Autodesk Inventor part; units mm, degrees
ref_plane "YZ Plane" through (0, 0, 0) normal (1, 0, 0) x (0, 1, 0)
ref_plane "XZ Plane" through (0, 0, 0) normal (0, 1, 0) x (-1, 0, 0)
ref_plane "XY Plane" through (0, 0, 0) normal (0, 0, 1) x (1, 0, 0)
sketch "Boceto1" plane through (0, 0, 0) normal (0, 1, 0) x (-1, 0, 0)
  line L0 (50, 50) -> (-50, 50)
  line L1 (-50, 50) -> (-50, -50)
  line L2 (-50, -50) -> (50, -50)
  line L3 (50, -50) -> (50, 50)
  line L4 (50, 50) -> (-50, -50) construction
  line L5 (-50, 50) -> (50, -50) construction
  point P0 (0, 0)
  dimension "d0" = 100
  dimension "d1" = 100
extrude "Extrusión1" add sketch "Boceto1" along normal blind 10
sketch "Boceto2" plane through (0, 10, 0) normal (0, 1, 0) x (1, 0, 0)
  line L0 (32.5, -35) -> (-32.5, -35)
  line L1 (-32.5, -35) -> (-32.5, -10)
  line L2 (-32.5, -10) -> (32.5, -10)
  line L3 (32.5, -10) -> (32.5, -35)
  line L4 (0, 0) -> (-40.0762, 0)
  line L5 (32.5, 35) -> (-32.5, 35)
  line L6 (-32.5, 35) -> (-32.5, 10)
  line L7 (-32.5, 10) -> (32.5, 10)
  line L8 (32.5, 10) -> (32.5, 35)
  dimension "d4" = 25
  dimension "d5" = 65
  dimension "d6" = 10
  dimension "d7" = 32.5
  dimension "d8" = 10
extrude "Extrusión2" add sketch "Boceto2" along normal blind 80
sketch "Boceto3" plane through (-32.5, 10, 35) normal (0, 0, 1) x (1, 0, 0)
  circle A0 centre (32.5, 55) radius 8.5
  line L0 (0, 0) -> (0, 80)
  line L1 (0, 80) -> (65, 80)
  point P0 (32.5, -10)
  dimension "d11" = 17
  dimension "d12" = 32.5
  dimension "d13" = 25
extrude "Extrusión3" cut sketch "Boceto3" against normal blind 80
fillet "Empalme1" radius 32.5 4 edges at (-32.5, 90, 22.5) (32.5, 90, 22.5) (32.5, 90, -22.5) (-32.5, 90, -22.5)
properties part number "03_10 soporte02" material "Acero ASTM A36"
Part model, mm, in its own coordinate system. A direction names the side the tool comes from. Coordinates: 2 decimals unless noted, no trailing zeros. Loops run counter-clockwise (first coordinate to the right, second up) from the corner with the lowest first, then second, coordinate; pieces in that order, holes last. Notation, with made-up numbers: (-22.75, -22.75) -> (27.25, -22.75) arc R25 cw to (27.25, 6.25) -> close; hole circle Ø1 at (-5.75, 70.5). An arc over 180 degrees is marked (long way). Use a Markdown table: item, result. Add a question column.
Item 1: Probe probe 1 along Z at (x, y) = (6, 17); probe 2 along Y at (x, z) = (0, 16.25); probe 3 along X at (y, z) = (47.5, 22). List the from-to ranges inside material, lowest first.
Item 2: Band-saw the part on D-D on x = -34. Write the cut outline in (y, z), plus the area to 3 significant figures.
Item 3: Flat gauge pins, fed straight in: P1, Ø6, axis at y = 46, z = 34.5, coming from the -X side; P2, Ø12, axis at x = 27.5, z = -35.5, coming from the +Y side; P3, Ø3, axis at x = 31.5, z = 4.5, coming from the +Y side. Where does each tip first touch, or does it go through?
Item 4: Pull direction Z, two halves, no side cores. Call faces 1 (the flat face through (0, 49, -10)), 2 (the flat face through (0, 49, 10)), 3 (the cylindrical face through (-23.23, 80.23, 22.32)), 4 (the flat face through (0, 49, 35)): +Z half, -Z half, draft (parallel to the pull), parting line (faces both ways), or undercut.
Item 5: Which spindle directions (+Z, -Z, +X, -X, +Y, -Y) get a long thin tool onto all of the face, cutting with end or side? Do faces 5 (the flat face through (32.5, 33, 22)), 6 (the flat face through (1, 10, 1)), 7 (the flat face through (-32.5, 33, 23)). Say none if no direction does.
Item 6: Band-saw the part on A-A on y = 16.5. Write the cut outline in (x, z), plus the area to 3 significant figures.
Item 7: Band-saw the part on C-C on y = 65. Write the cut outline in (x, z), plus the area to 3 significant figures.
Geometry says:
| question | item | result |
|---|---|---|
| 1 | probe 1 | -35 to -10, 10 to 35 |
| 1 | probe 2 | 0 to 56.5, 73.5 to 90 |
| 1 | probe 3 | -32.5 to 32.5 |
| 2 | outline | (0, -50) -> (10, -50) -> (10, 50) -> (0, 50) -> close |
| 2 | area | 1,000 mm² |
| 3 | P1 | x = -32.5 |
| 3 | P2 | y = 81.85 |
| 3 | P3 | y = 10 |
| 4 | face 1 | undercut |
| 4 | face 2 | undercut |
| 4 | face 3 | draft |
| 4 | face 4 | +Z half |
| 5 | face 5 | +Z, -Z, +X, +Y |
| 5 | face 6 | +Y |
| 5 | face 7 | +Z, -Z, -X, +Y |
| 6 | outline | (-32.5, -35) -> (32.5, -35) -> (32.5, -10) -> (-32.5, -10) -> close; (-32.5, 10) -> (32.5, 10) -> (32.5, 35) -> (-32.5, 35) -> close |
| 6 | area | 3,250 mm² |
| 7 | outline | (-31.62, -35) -> (-8.5, -35) -> (-8.5, -10) -> (-31.62, -10) -> close; (-31.62, 10) -> (-8.5, 10) -> (-8.5, 35) -> (-31.62, 35) -> close; (8.5, -35) -> (31.62, -35) -> (31.62, -10) -> (8.5, -10) -> close; (8.5, 10) -> (31.62, 10) -> (31.62, 35) -> (8.5, 35) -> close |
| 7 | area | 2,310 mm² |
